```python
from build123d import *
from OCP.BRepFilletAPI import BRepFilletAPI_MakeChamfer

# Parameters (mm, degrees)
SKETCH1_R           = 57.5
BOSS_EXTRUDE1_DEPTH = 230.197861
SKETCH2_R           = 46.429396427
CUT_EXTRUDE1_DEPTH  = 245.138393558
CHAMFER1_SIZE       = 3.935281
CHAMFER1_SIZE2      = 3.707563


with BuildPart() as part:
    # Sketch1 → Boss-Extrude1 (new body)
    with BuildSketch(Plane(origin=(0, 0, 0), x_dir=(1, 0, 0), z_dir=(0, 1, 0))):
        with Locations(Location((0, 0, 0), (0, 0, 270))):
            Circle(SKETCH1_R)
    extrude(amount=BOSS_EXTRUDE1_DEPTH)

    # Sketch2 → Cut-Extrude1 (cut, through all)
    with BuildSketch(Plane(origin=(0, 0, 0), x_dir=(1, 0, 0), z_dir=(0, 1, 0))):
        with Locations(Location((0, 0, 0), (0, 0, 270))):
            Circle(SKETCH2_R)
    extrude(amount=CUT_EXTRUDE1_DEPTH, mode=Mode.SUBTRACT)

    # Chamfer1: one chamfer whose edges measure the first distance from different faces: ONE call of the kernel's chamfer builder (chamfer() names one face for all edges)
    chamfer1_edges_1 = [part.edges().sort_by_distance(p)[0] for p in [
        (0, 0, -57.5),
    ]]
    chamfer1_side_1 = [part.faces().sort_by_distance(p)[0] for p in [
        (0, 115.0989305, -57.5),
    ]]
    chamfer1_edges_2 = [part.edges().sort_by_distance(p)[0] for p in [
        (0, 230.197861, -57.5),
    ]]
    chamfer1_side_2 = [part.faces().sort_by_distance(p)[0] for p in [
        (0, 230.197861, -55.873654403),
    ]]
    chamfer1_edges_3 = [part.edges().sort_by_distance(p)[0] for p in [
        (0, 0, -46.429396427),
    ]]
    chamfer1_side_3 = [part.faces().sort_by_distance(p)[0] for p in [
        (0, 0, -55.873654403),
    ]]
    chamfer1_edges_4 = [part.edges().sort_by_distance(p)[0] for p in [
        (0, 230.197861, -46.429396427),
    ]]
    chamfer1_side_4 = [part.faces().sort_by_distance(p)[0] for p in [
        (0, 115.0989305, -46.429396427),
    ]]
    chamfer1 = BRepFilletAPI_MakeChamfer(part.part.solid().wrapped)
    for e in chamfer1_edges_1:
        chamfer1.Add(CHAMFER1_SIZE, CHAMFER1_SIZE2, e.wrapped, chamfer1_side_1[0].wrapped)  # the first distance lies on this face
    for e in chamfer1_edges_2:
        chamfer1.Add(CHAMFER1_SIZE, CHAMFER1_SIZE2, e.wrapped, chamfer1_side_2[0].wrapped)  # the first distance lies on this face
    for e in chamfer1_edges_3:
        chamfer1.Add(CHAMFER1_SIZE, CHAMFER1_SIZE2, e.wrapped, chamfer1_side_3[0].wrapped)  # the first distance lies on this face
    for e in chamfer1_edges_4:
        chamfer1.Add(CHAMFER1_SIZE, CHAMFER1_SIZE2, e.wrapped, chamfer1_side_4[0].wrapped)  # the first distance lies on this face
    add(Compound.cast(chamfer1.Shape()), mode=Mode.REPLACE)


solid = part.part
```
Work out the finished part from the listing and answer in its coordinate system (mm). Coordinates: 2 decimals unless noted, no trailing zeros. Loops run counter-clockwise (first coordinate to the right, second up) from the corner with the lowest first, then second, coordinate; pieces in that order, holes last. Notation, with made-up numbers: M -24,46.5 L -1,46.5 A5 ccw -1,50.5 Z; hole C 80,13.25 d11. An arc over 180 degrees is marked long. Use CSV: the item, a comma, the result in double quotes. Start each with the question number.
(1) Find section A-A, the plane x = 0. Give the vertices of the cut face in (y, z), then the cut area to 3 significant figures.
(2) Given pin 1 Ø10 at (y, z) = (86.5, -9) entering from +X; pin 2 Ø10 at (y, z) = (127, 26) entering from +X; pin 3 Ø5 at (y, z) = (206.5, -23) entering from -X, each flat-ended and moving along its own axis, determine where each tip first touches the part or whether it passes through.
(3) Consider line 1 (X direction, y = 69, z = 0); line 2 (X direction, y = 96.5, z = 27.5). Determine where each line is inside the solid, lowest interval first.
(4) Find section B-B, the plane z = 0. Give the vertices of the cut face in (x, y).
(5) Find section C-C, the plane y = 108.5. Give the vertices of the cut face in (x, z), then the cut area to 3 significant figures.
(6) For a pull along X with two mould halves and no side action, classify faces 1 (the face through (-56.133, 113.655, -12.465)), 2 (the face through (-16, 0, -48)), 3 (the face through (39.15, 113.43, 24.96)), 4 (the face through (-45.51, 3.53, -10.11)) as +X half, -X half, draft (parallel to the pull), parting line (faces both ways), or undercut.
Recorded:
1,outline,"M 0,-53.79 L 3.94,-57.5 L 226.49,-57.5 L 230.2,-53.56 L 230.2,-50.14 L 226.26,-46.43 L 3.71,-46.43 L 0,-50.36 Z; M 0,50.36 L 3.71,46.43 L 226.26,46.43 L 230.2,50.14 L 230.2,53.56 L 226.49,57.5 L 3.94,57.5 L 0,53.79 Z"
1,area,"5,040 mm^2"
2,pin 1,"stops at x = 57.36"
2,pin 2,"stops at x = 53.53"
2,pin 3,"stops at x = -53.72"
3,line 1,"x = -57.5 to -46.43, 46.43 to 57.5"
3,line 2,"x = -50.5 to -37.41, 37.41 to 50.5"
4,outline,"M -57.5,3.94 L -53.79,0 L -50.36,0 L -46.43,3.71 L -46.43,226.26 L -50.14,230.2 L -53.56,230.2 L -57.5,226.49 Z; M 46.43,3.71 L 50.36,0 L 53.79,0 L 57.5,3.94 L 57.5,226.49 L 53.56,230.2 L 50.14,230.2 L 46.43,226.26 Z"
5,outline,"C 0,0 d115; hole C 0,0 d92.86"
5,area,"3,610 mm^2"
6,face 1,"parting line"
6,face 2,"draft"
6,face 3,"undercut"
6,face 4,"undercut"
